Check sheet for the modelled part. Datum: model origin and axes. Units: mm. A direction names the side the tool comes from. Round coordinates to 2 decimals unless told otherwise and drop trailing zeros. Write each loop counter-clockwise with the first axis right and the second up, starting at its lowest first coordinate (ties: lowest second). Pieces come first, ordered by that corner, then holes.
Item 1: Section check B-B, the plane y = 0. Record the cut outline in (x, z), plus the area to 3 significant figures.
Item 2: Section check A-A, the plane z = 0. State how many separate pieces and enclosed holes the cut face has, plus the area to 3 significant figures.
Item 3: Section check C-C, the plane x = 40.5. Record the cut outline in (y, z), plus the area to 3 significant figures.
Item 4: Set-up check for faces 4 (the cylindrical face through (6.08, -32.88, 39.2)), 5 (the flat face through (25, -8, -24)): record each of +Z, -Z, +X, -X, +Y, -Y from which the full face is reachable in a straight line by a thin tool's end or side.
Item 5: Depth check by flat-ended pin: pin 1 (1 mm diameter, centred on x = 20, z = -34, fed in from +Y); pin 2 (12 mm diameter, centred on x = 14, y = 39, fed in from -Z); pin 3 (1 mm diameter, centred on y = 42, z = 26.5, fed in from +X). Enter the tip coordinate at first touch or a pass-through.
Item 6: Material ranges on line 1 along Y through (x, z) = (7, 50.5); line 2 along Y through (x, z) = (10, -46.5); line 3 along Z through (x, y) = (6, -27), recorded low to high.
Item 7: Release check for a two-part mould opening along Y. For faces 1 (the cylindrical face through (6.08, 20.13, 54.39)), 2 (the flat face through (12, 31, -31)), 3 (the cylindrical face through (30.76, -1.76, -39.96)) record: pulls with the +Y half, pulls with the -Y half, needs draft (parallel to the pull), parting line crosses it, or undercut.
from build123d import *

# Parameters (mm, degrees)
SKETCH_2_W               = 12
SKETCH_2_H               = 10
PATTERN_CIRCULAR_1_COUNT = 6
FILLET_1_R               = 2
CHAMFER_1_SIZE           = 2
CHAMFER_3_SIZE           = 3
CHAMFER_3_SIZE2          = 5.196152423


with BuildPart() as part:
    # Эскиз1 → Повернуть1 (revolve)
    with BuildSketch(Plane.XY, mode=Mode.PRIVATE) as revolve_1_sk:
        Polygon((0, 35), (25, 35), (25, 25), (50, 25), (50, 40), (12, 40), (12, 75), (0, 75), align=None)
    revolve(revolve_1_sk.sketch.rotate(Axis((0, 0, 0), (1, 0, 0)), 90), axis=Axis((0, 0, 0), (1, 0, 0)))

    # Эскиз2 → Вырез-Повернуть1 (revolve, cut)
    with BuildSketch(Plane.XY, mode=Mode.PRIVATE) as cut_revolve_1_sk:
        with Locations((6, 60)):
            Rectangle(SKETCH_2_W, SKETCH_2_H)
    cut_revolve_1 = revolve(cut_revolve_1_sk.sketch.rotate(Axis((12, 55, 0), (1, 0, 0)), 180), axis=Axis((12, 55, 0), (1, 0, 0)), mode=Mode.SUBTRACT)

    # Круговой массив1: Вырез-Повернуть1 ×6 about axis
    pattern_circular_1_axis = Axis((0, 0, 0), (1, 0, 0))
    for i in range(1, PATTERN_CIRCULAR_1_COUNT):
        add(cut_revolve_1.rotate(pattern_circular_1_axis, i * 360 / PATTERN_CIRCULAR_1_COUNT), mode=Mode.SUBTRACT)

    # Скругление1
    fillet_1_edges = [part.edges().sort_by_distance(p)[0] for p in [
        (0, 0, -75),
        (12, 0, -75),
        (12, 0, -40),
    ]]
    fillet(fillet_1_edges, radius=FILLET_1_R)

    # Фаска1
    chamfer_1_edges = [part.edges().sort_by_distance(p)[0] for p in [
        (50, 0, -40),
    ]]
    chamfer(chamfer_1_edges, length=CHAMFER_1_SIZE)

    # Фаска3
    chamfer_3_edges = [part.edges().sort_by_distance(p)[0] for p in [
        (50, 0, -25),
    ]]
    chamfer_3_side = [part.faces().sort_by_distance(p)[0] for p in [
        (37.5, 0, -25),
    ]]
    chamfer(chamfer_3_edges, length=CHAMFER_3_SIZE, length2=CHAMFER_3_SIZE2, reference=chamfer_3_side[0])


solid = part.part
Values found:
1. outline: (0, -73) arc R2 ccw to (2, -75) - (10, -75) arc R2 ccw to (12, -73) - (12, -42) arc R2 cw to (14, -40) - (48, -40) - (50, -38) - (50, -30.2) - (47, -25) - (25, -25) - (25, -35) - (0, -35) - close; (0, 35) - (25, 35) - (25, 25) - (47, 25) - (50, 30.2) - (50, 38) - (48, 40) - (14, 40) arc R2 cw to (12, 42) - (12, 73) arc R2 ccw to (10, 75) - (2, 75) arc R2 ccw to (0, 73) - close
1. area: 1,820 mm2
2. separate pieces: 4
2. enclosed holes: 0
2. area: 1,340 mm2
3. outline: circle Ø80 at (0, 0); hole circle Ø50 at (0, 0)
3. area: 3,060 mm2
4. face 4: +X, -X
4. face 5: -X
5. pin 1: stops at y = 21.86
5. pin 2: stops at z = -66.72
5. pin 3: stops at x = 12
6. line 1: y = -55.45 to -37.08, -17.92 to 17.92, 37.08 to 55.45
6. line 2: y = -58.85 to -37.44, -17.56 to 17.56, 37.44 to 58.85
6. line 3: z = -69.97 to -57.62, -37.64 to -22.27, 22.27 to 37.64, 57.62 to 69.97
7. face 1: undercut
7. face 2: needs draft
7. face 3: parting line crosses it
